Here's the drawing with two shaded views (mm, measured from the low corner). I have some questions. A direction names the side the tool comes from. Coordinates: 2 decimals unless noted, no trailing zeros. Loops run counter-clockwise (first coordinate to the right, second up) from the corner with the lowest first, then second, coordinate; pieces in that order, holes last. Notation, with made-up numbers: (-2.5, -27.75) - (7.5, -27.75) arc R30 ccw to (7.5, -2.75) - close; hole circle Ø3 at (-4.75, -35). An arc over 180 degrees is marked (long way). Use a Markdown table: item, result.
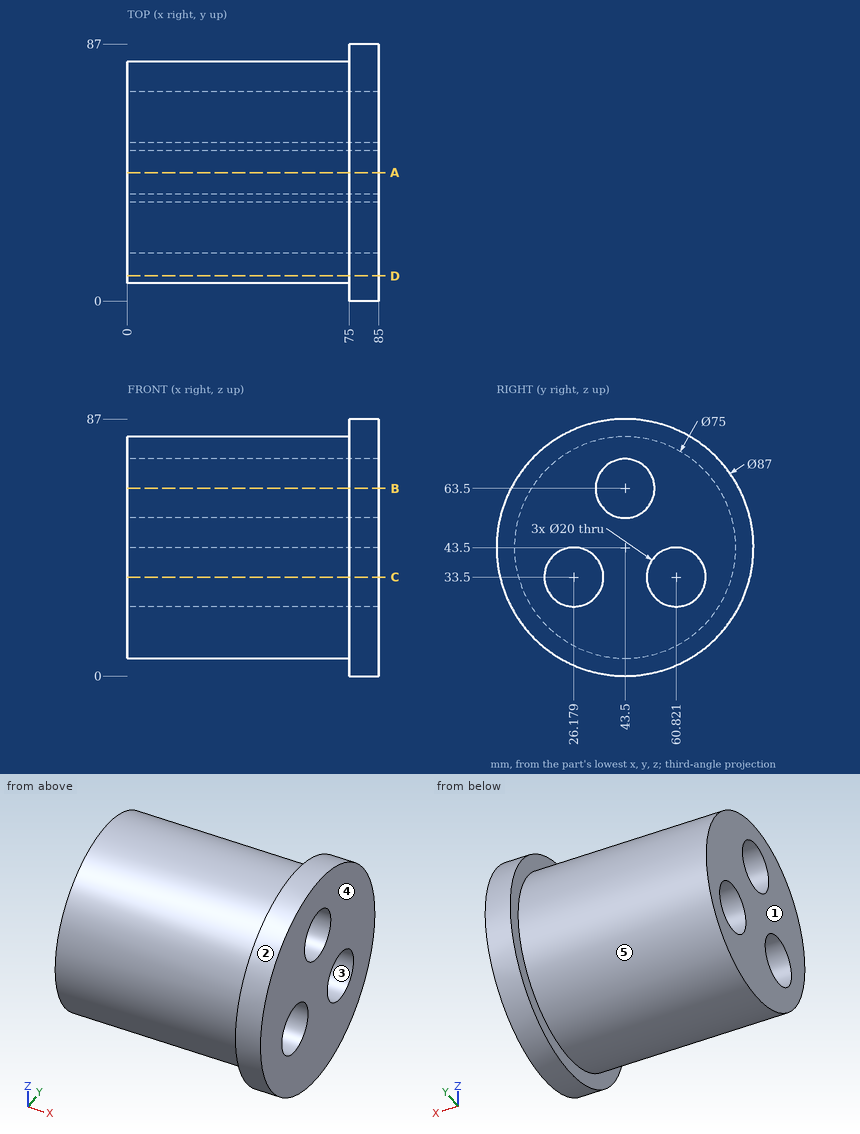
Q1. I want a section at C-C, the plane z = 33.5. Write out the boundary of the cut face in (x, y) (1 decimal).
Check values:
| item | result |
|---|---|
| outline | (0, 7.4) - (75, 7.4) - (75, 1.2) - (85, 1.2) - (85, 16.2) - (0, 16.2) - close; (0, 36.2) - (85, 36.2) - (85, 50.8) - (0, 50.8) - close; (0, 70.8) - (85, 70.8) - (85, 85.8) - (75, 85.8) - (75, 79.6) - (0, 79.6) - close |
Q2. Will these pins go through, and if not, where does the flat tip stop? P1, Ø10, axis at x = 12, z = 20, coming from the +Y side; P2, Ø1.5, axis at x = 14, z = 41.5, coming from the -Y side; P3, Ø2, axis at x = 67, z = 19.5, coming from the -Y side.
Check values:
| item | result |
|---|---|
| P1 | y = 76.12 |
| P2 | y = 6.02 |
| P3 | y = 13.88 |
Q3. I want a section at A-A, the plane y = 43.5. Write out the boundary of the cut face in (x, z).
Check values:
| item | result |
|---|---|
| outline | (0, 6) - (75, 6) - (75, 0) - (85, 0) - (85, 53.5) - (0, 53.5) - close; (0, 73.5) - (85, 73.5) - (85, 87) - (75, 87) - (75, 81) - (0, 81) - close |
Q4. I want a section at D-D, the plane y = 8.5. Write out the boundary of the cut face in (x, z), then the cut area to 3 significant figures.
Check values:
| item | result |
|---|---|
| outline | (0, 30.04) - (75, 30.04) - (75, 17.67) - (85, 17.67) - (85, 69.33) - (75, 69.33) - (75, 56.96) - (0, 56.96) - close |
| area | 2,540 mm^2 |
Q5. Which directions (+Z, -Z, +X, -X, +Y, -Y) give clear straight access to the entire face, cutting with the end or side of a thin tool? Please do the marked faces 4 and 5.
Check values:
| item | result |
|---|---|
| face 4 | +Z, -Z, +X, +Y, -Y |
| face 5 | -X |
Q6. I want a section at B-B, the plane z = 63.5. Write out the boundary of the cut face in (x, y), then the cut area to 3 significant figures.
Check values:
| item | result |
|---|---|
| outline | (0, 11.78) - (75, 11.78) - (75, 4.87) - (85, 4.87) - (85, 33.5) - (0, 33.5) - close; (0, 53.5) - (85, 53.5) - (85, 82.13) - (75, 82.13) - (75, 75.22) - (0, 75.22) - close |
| area | 3,830 mm^2 |
Q7. Please list where these lines run through material, in increasing order: L1, parallel to Y at x = 72.5, z = 37; L2, parallel to Y at x = 18.5, z = 33.5; L3, parallel to Y at x = 80.5, z = 65.5 (1 decimal). Write a range as from..to.
Check values:
| item | result |
|---|---|
| L1 | 6.57..16.81, 35.55..51.45, 70.19..80.43 |
| L2 | 7.36..16.18, 36.18..50.82, 70.82..79.64 |
| L3 | 6..33.7, 53.3..81 |
Q8. If we mould it in two halves opening along Y, with no side actions, what happens to the marked faces 1, 2 and 3? For each: pulls with the +Y half, pulls with the -Y half, needs draft (parallel to the pull), parting line crosses it, or undercut.
Check values:
| item | result |
|---|---|
| face 1 | needs draft |
| face 2 | parting line crosses it |
| face 3 | undercut |
